```python
from build123d import *

# Parameters (mm, degrees)
BOSS_EXTRUDE1_DEPTH = 5.08
SKETCH3_R           = 3.302
BOSS_EXTRUDE2_DEPTH = 76.2


with BuildPart() as part:
    # Sketch2 → Boss-Extrude1 (new body)
    with BuildSketch(Plane(origin=(0, 0, 0), x_dir=(0, 0, -1), z_dir=(1, 0, 0))):
        Polygon((0, -4.399409051), (3.81, -2.199704526), (3.81, 2.199704526), (0, 4.399409051), (-3.81, 2.199704526), (-3.81, -2.199704526), align=None)
    extrude(amount=BOSS_EXTRUDE1_DEPTH)

    # Sketch3 → Boss-Extrude2 (add)
    with BuildSketch(Plane(origin=(5.08, 0, 0), x_dir=(0, 0, -1), z_dir=(1, 0, 0))):
        with Locations(Location((0, 0, 0), (0, 0, 180))):
            Circle(SKETCH3_R)
    extrude(amount=BOSS_EXTRUDE2_DEPTH)

    # Sketch4 → Cut-Revolve1 (revolve, cut)
    with BuildSketch(Plane.XY, mode=Mode.PRIVATE) as cut_revolve1_sk:
        Polygon((5.08, 4.399409051), (0.762, 4.399409051), (0, 3.637409051), (0, 2.199704526), (-1.146784512, 2.199704526), (-1.146784512, 5.580945805), (5.08, 5.580945805), align=None)
    revolve(cut_revolve1_sk.sketch.rotate(Axis((0, 0, 0), (1, 0, 0)), 300.000000093), axis=Axis((0, 0, 0), (1, 0, 0)), mode=Mode.SUBTRACT)


solid = part.part
```
Design review of the part built by this model. Coordinates are the model's own, in mm. A direction names the side the tool comes from. Coordinates: 2 decimals unless noted, no trailing zeros. Loops run counter-clockwise (first coordinate to the right, second up) from the corner with the lowest first, then second, coordinate; pieces in that order, holes last. Notation, with made-up numbers: M 56.5,26 L 115.5,26 A29 ccw 115.5,55 Z; hole C -13.75,48 d7. An arc over 180 degrees is marked long. One line per question, with ' | ' between items.
(1) We need section A-A (y = 0). Give the boundary of the cut face in (x, z), and give its area (3 significant figures).
Filled in:
outline: M 0,-3.64 L 0.17,-3.81 L 5.08,-3.81 L 5.08,-3.3 L 81.28,-3.3 L 81.28,3.3 L 5.08,3.3 L 5.08,3.81 L 0.17,3.81 L 0,3.64 Z | area: 542 mm^2
(2) Wall thickness on probe 1 along X at (y, z) = (-1, -3.5); probe 2 along X at (y, z) = (3.5, 1.5); probe 3 along Z at (x, y) = (28.5, 3): over which ranges is each line inside the solid? List them lowest first.
Filled in:
probe 1: x = 0 to 5.08 | probe 2: x = 0.17 to 5.08 | probe 3: z = -1.38 to 1.38
(3) For pin 1 Ø3 at (x, z) = (41.5, 2.5) entering from -Y; pin 2 Ø3 at (x, z) = (44.5, 2.5) entering from +Y, all flat-tipped, find the tip position at first contact; note any pin that passes through.
Filled in:
pin 1: stops at y = -3.15 | pin 2: stops at y = 3.15
(4) Machinability: for faces 1 (the face through (5.08, -2, -3)), 2 (the face through (81.28, 0, 0)), which of the approach directions +Z, -Z, +X, -X, +Y, -Y give a long, thin tool a straight path to every point of the face, cutting with its end or side? Answer none if there is none.
Filled in:
face 1: +X | face 2: +Z, -Z, +X, +Y, -Y
(5) We need section B-B (x = 62.5). Give the boundary of the cut face in (y, z), and give its area (3 significant figures).
Filled in:
outline: C 0,0 d6.6 | area: 34.3 mm^2
